Design review of the part built by this model. Coordinates are the model's own, in mm. A direction names the side the tool comes from. Round coordinates to 2 decimals unless told otherwise and drop trailing zeros. Loops run counter-clockwise (first coordinate to the right, second up) from the corner with the lowest first, then second, coordinate; pieces in that order, holes last. Notation, with made-up numbers: M 70,24 L 83,24 A9 cw 83,33 Z; hole C 23.25,6.5 d2. An arc over 180 degrees is marked long. Use a Markdown table: item, result.
from build123d import *

# Parameters (mm, degrees)
SKETCH001_W  = 119
SKETCH001_H  = 54
PAD_DEPTH    = 1
SKETCH_R     = 4
PAD001_DEPTH = 132
SKETCH002_W  = 115.57
SKETCH002_H  = 135.89
POCKET_DEPTH = 50
PAD002_DEPTH = 1
SKETCH003_R  = 1.4
PAD003_DEPTH = 4


with BuildPart() as part:
    # Sketch001 → Pad (new body)
    with BuildSketch(Plane.XY):
        Rectangle(SKETCH001_W, SKETCH001_H)
    extrude(amount=-PAD_DEPTH)

    # Sketch → Pad001 (join)
    with BuildSketch(Plane.XY):
        with Locations((-52.5, 20)):
            Circle(SKETCH_R)
        with Locations((52.5, 20)):
            Circle(SKETCH_R)
        with Locations((52.5, -20)):
            Circle(SKETCH_R)
        with Locations((-52.5, -20)):
            Circle(SKETCH_R)
    extrude(amount=PAD001_DEPTH)

    # Sketch002 (on DatumPlane) → Pocket (cut)
    with BuildSketch(Plane(origin=(0, -27, 0), x_dir=(1, 0, 0), z_dir=(0, -0.939693, 0.34202))):
        with Locations((0, 72.945)):
            Rectangle(SKETCH002_W, SKETCH002_H)
    extrude(amount=POCKET_DEPTH, mode=Mode.SUBTRACT)

    # Sketch002 (on DatumPlane) → Pad002 (join)
    with BuildSketch(Plane(origin=(0, -27, 0), x_dir=(1, 0, 0), z_dir=(0, -0.939693, 0.34202))):
        with Locations((0, 72.945)):
            Rectangle(SKETCH002_W, SKETCH002_H)
    extrude(amount=PAD002_DEPTH)

    # Sketch003 (on DatumPlane) → Pad003 (join)
    with BuildSketch(Plane(origin=(0, -27, 0), x_dir=(1, 0, 0), z_dir=(0, -0.939693, 0.34202))):
        with Locations((-54.61, 137.715)):
            Circle(SKETCH003_R)
        with Locations((54.61, 137.715)):
            Circle(SKETCH003_R)
        with Locations((54.61, 8.175)):
            Circle(SKETCH003_R)
        with Locations((-54.61, 8.175)):
            Circle(SKETCH003_R)
    extrude(amount=PAD003_DEPTH)


solid = part.part
1. The part is to be moulded in two halves that separate along Z. For faces 3 (the face through (-53.021, 23.966, 65.076)), 4 (the face through (57.785, -3, 68)), 5 (the face through (-1, 0, -1)), 6 (the face through (-53.275, 17.916, 130.653)), say which applies: pulls with the +Z half, pulls with the -Z half, needs draft (parallel to the pull), parting line crosses it, or undercut.
Check values:
| item | result |
|---|---|
| face 3 | undercut |
| face 4 | needs draft |
| face 5 | pulls with the -Z half |
| face 6 | undercut |
2. Insertion check: pin 1 (3.5 mm diameter, centred on x = -53, y = 22.5, fed in from +Z); pin 2 (6 mm diameter, centred on x = -24.5, z = 105.5, fed in from -Y); pin 3 (1 mm diameter, centred on x = 14.5, z = 91, fed in from +Y); pin 4 (8 mm diameter, centred on y = 8.5, z = 47.5, fed in from -X). Each pin has a flat end and moves straight along its axis. Give the tip position at first contact, or say it passes through.
Check values:
| item | result |
|---|---|
| pin 1 | stops at z = 132.55 |
| pin 2 | stops at y = 9.24 |
| pin 3 | stops at y = 6.3 |
| pin 4 | passes through |
3. Take a section at C-C on z = 38.5. Give the boundary of the cut face in (x, y) (3 decimals), and give its area (3 significant figures).
Check values:
| item | result |
|---|---|
| outline | M -57.785,-14.051 L 57.785,-14.051 L 57.785,-12.987 L -57.785,-12.987 Z; C -52.5,20 d8; C 52.5,20 d8 |
| area | 224 mm² |
4. Take a section at A-A on x = 36.5. Give the boundary of the cut face in (y, z), and give its area (3 significant figures).
Check values:
| item | result |
|---|---|
| outline | M -27,-1 L 27,-1 L 27,0 L -27,0 Z; M -26.23,5.04 L -25.29,4.7 L 21.19,132.39 L 20.25,132.74 Z |
| area | 190 mm² |
5. Wall thickness on line 1 along Y through (x, z) = (-51, 69.5); line 2 along Y through (x, z) = (55.5, 82); line 3 along X through (y, z) = (16.5, 50): over which ranges is each line inside the solid? List them lowest first. Write a range as from..to.
Check values:
| item | result |
|---|---|
| line 1 | y = -2.77..-1.7, 16.29..23.71 |
| line 2 | y = 1.78..2.85, 17.35..22.65 |
| line 3 | x = -54.44..-50.56, 50.56..54.44 |
6. Machinability: for faces 1 (the face through (-57.785, -3, 68)), 2 (the face through (-1, 0, 0)), which of the approach directions +Z, -Z, +X, -X, +Y, -Y give a long, thin tool a straight path to every point of the face, cutting with its end or side? Answer none if there is none.
Check values:
| item | result |
|---|---|
| face 1 | +Z, -X, +Y, -Y |
| face 2 | none |
7. Take a section at B-B on y = -8. Give the boundary of the cut face in (x, z) (3 decimals), and give its area (3 significant figures).
Check values:
| item | result |
|---|---|
| outline | M -59.5,-1 L 59.5,-1 L 59.5,0 L -59.5,0 Z; M -57.785,52.202 L 57.785,52.202 L 57.785,55.126 L -57.785,55.126 Z |
| area | 457 mm² |
